Verification items for the finished model (mm, model axes). Give positions to 0.01 mm unless a question says otherwise; leave off trailing zeros. Loops run counter-clockwise (first coordinate to the right, second up) from the corner with the lowest first, then second, coordinate; pieces in that order, holes last. Notation, with made-up numbers: (55, 70) - (80, 70) arc R12 ccw to (80, 76) - close; hole circle Ø8 at (59, 43). An arc over 180 degrees is marked (long way). Answer in a Markdown table with one row per item.
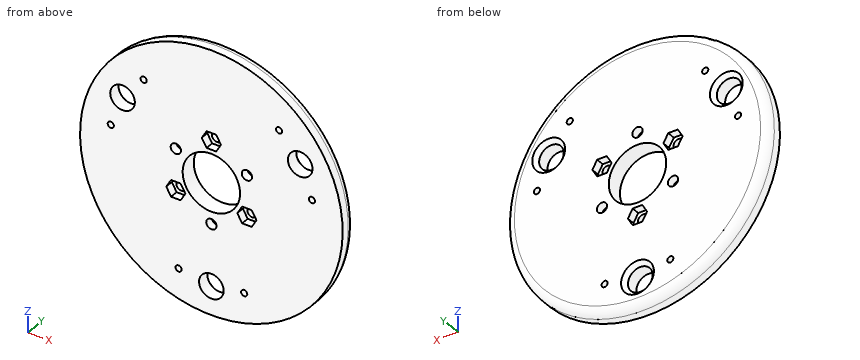
```python
from build123d import *

# Parameters (mm, degrees)
SKETCH_1_R          = 32
SKETCH_1_R_2        = 7
SKETCH_1_R_3        = 3
EXTRUDE_1_DEPTH     = 4
FILLET_1_R          = 2
SKETCH_2_R          = 1.25
CUT_EXTRUDE_1_DEPTH = 46.431266766
CUT_EXTRUDE_2_DEPTH = 2
CUT_EXTRUDE_3_DEPTH = 2
CHAMFER_1_SIZE      = 1
SKETCH_5_R          = 0.75
CUT_EXTRUDE_4_DEPTH = 46.431266766


with BuildPart() as part:
    # Эскиз1 → Бобышка-Вытянуть1 (new body)
    with BuildSketch(Plane(origin=(0, 0, 0), x_dir=(1, 0, 0), z_dir=(0, 1, 0))):
        with Locations(Location((0, 0, 0), (0, 0, 270))):
            Circle(SKETCH_1_R)
        with Locations(Location((0, 0, 0), (0, 0, 270))):
            Circle(SKETCH_1_R_2, mode=Mode.SUBTRACT)
        with Locations(Location((0, 25, 0), (0, 0, 270))):
            Circle(SKETCH_1_R_3, mode=Mode.SUBTRACT)
        with Locations(Location((21.650635095, -12.5, 0), (0, 0, 270))):
            Circle(SKETCH_1_R_3, mode=Mode.SUBTRACT)
        with Locations(Location((-21.650635095, -12.5, 0), (0, 0, 270))):
            Circle(SKETCH_1_R_3, mode=Mode.SUBTRACT)
    extrude(amount=EXTRUDE_1_DEPTH)

    # Скругление1
    fillet_1_edges = [part.edges().sort_by_distance(p)[0] for p in [
        (0, 4, -32),
    ]]
    fillet(fillet_1_edges, radius=FILLET_1_R)

    # Эскиз2 → Вырез-Вытянуть1 (cut, through all)
    with BuildSketch(Plane(origin=(0, 4, 0), x_dir=(1, 0, 0), z_dir=(0, 1, 0))):
        with Locations(Location((0, 10, 0), (0, 0, 270))):
            Circle(SKETCH_2_R)
        with Locations(Location((8.660254038, 5, 0), (0, 0, 270))):
            Circle(SKETCH_2_R)
        with Locations(Location((8.660254038, -5, 0), (0, 0, 270))):
            Circle(SKETCH_2_R)
        with Locations(Location((0, -10, 0), (0, 0, 270))):
            Circle(SKETCH_2_R)
        with Locations(Location((-8.660254038, -5, 0), (0, 0, 270))):
            Circle(SKETCH_2_R)
        with Locations(Location((-8.660254038, 5, 0), (0, 0, 270))):
            Circle(SKETCH_2_R)
    extrude(amount=-CUT_EXTRUDE_1_DEPTH, mode=Mode.SUBTRACT)

    # Эскиз3 → Вырез-Вытянуть2 (cut)
    with BuildSketch(Plane(origin=(0, 4, 0), x_dir=(1, 0, 0), z_dir=(0, 1, 0))):
        Polygon((9.829388333, -7.025), (10.998522628, -5), (9.829388333, -2.975), (7.491119743, -2.975), (6.321985448, -5), (7.491119743, -7.025), align=None)
        Polygon((1.169134295, 7.975), (2.33826859, 10), (1.169134295, 12.025), (-1.169134295, 12.025), (-2.33826859, 10), (-1.169134295, 7.975), align=None)
        Polygon((-10.998522628, -5), (-9.829388333, -7.025), (-7.491119743, -7.025), (-6.321985448, -5), (-7.491119743, -2.975), (-9.829388333, -2.975), align=None)
    extrude(amount=-CUT_EXTRUDE_2_DEPTH, mode=Mode.SUBTRACT)

    # Эскиз4 → Вырез-Вытянуть3 (cut)
    with BuildSketch(Plane.XZ):
        Polygon((7.491119743, -7.025), (9.829388333, -7.025), (10.998522628, -5), (9.829388333, -2.975), (7.491119743, -2.975), (6.321985448, -5), align=None)
        Polygon((-1.169134295, 7.975), (1.169134295, 7.975), (2.33826859, 10), (1.169134295, 12.025), (-1.169134295, 12.025), (-2.33826859, 10), align=None)
        Polygon((-9.829388333, -2.975), (-10.998522628, -5), (-9.829388333, -7.025), (-7.491119743, -7.025), (-6.321985448, -5), (-7.491119743, -2.975), align=None)
    extrude(amount=-CUT_EXTRUDE_3_DEPTH, mode=Mode.SUBTRACT)

    # Фаска1
    chamfer_1_edges = [part.edges().sort_by_distance(p)[0] for p in [
        (21.650635095, 4, 9.5),
        (-21.650635095, 4, 9.5),
        (0, 4, -28),
    ]]
    chamfer(chamfer_1_edges, length=CHAMFER_1_SIZE)

    # Эскиз5 → Вырез-Вытянуть4 (cut, through all)
    with BuildSketch(Plane(origin=(0, 4, 0), x_dir=(1, 0, 0), z_dir=(0, 1, 0))):
        with Locations(Location((8, 23.685438565, 0), (0, 0, 270))):
            Circle(SKETCH_5_R)
        with Locations(Location((-8, 23.685438565, 0), (0, 0, 270))):
            Circle(SKETCH_5_R)
        with Locations(Location((24.512191497, -4.914516052, 0), (0, 0, 270))):
            Circle(SKETCH_5_R)
        with Locations(Location((16.512191497, -18.770922513, 0), (0, 0, 270))):
            Circle(SKETCH_5_R)
        with Locations(Location((-16.512191497, -18.770922513, 0), (0, 0, 270))):
            Circle(SKETCH_5_R)
        with Locations(Location((-24.512191497, -4.914516052, 0), (0, 0, 270))):
            Circle(SKETCH_5_R)
    extrude(amount=-CUT_EXTRUDE_4_DEPTH, mode=Mode.SUBTRACT)


solid = part.part
```
Q1. Thickness scan on line 1 (X direction, y = 0.95, z = 10); line 2 (X direction, y = 0.95, z = 5); line 3 (X direction, y = 2.5, z = 10). Record the ranges inside material, lowest first.
Completed:
| item | result |
|---|---|
| line 1 | -30.4 to -23.31, -19.99 to -2.34, 2.34 to 19.99, 23.31 to 30.4 |
| line 2 | -31.61 to -25.26, -23.77 to -9.91, -7.41 to -4.9, 4.9 to 7.41, 9.91 to 23.77, 25.26 to 31.61 |
| line 3 | -30.33 to -23.31, -19.99 to -1.25, 1.25 to 19.99, 23.31 to 30.33 |
Q2. Sectioned sample at B-B (z = 0). Record the cut outline in (x, y), and give its area (3 significant figures).
Completed:
| item | result |
|---|---|
| outline | (-32, 0) - (-7, 0) - (-7, 4) - (-30, 4) arc R2 ccw to (-32, 2) - close; (7, 0) - (32, 0) - (32, 2) arc R2 ccw to (30, 4) - (7, 4) - close |
| area | 198 mm^2 |
Q3. Sectioned sample at A-A (x = 0). Give the number of separate pieces and of enclosed holes in the cut face, and give its area (3 significant figures).
Completed:
| item | result |
|---|---|
| separate pieces | 5 |
| enclosed holes | 0 |
| area | 147 mm^2 |
Q4. Go/stop test with flat-tipped pins: P1, Ø3, axis at x = 8.66, z = 5, coming from the -Y side; P2, Ø1.5, axis at y = 3, z = -24.5, coming from the -X side; P3, Ø0.6, axis at x = -9, y = 1.5, coming from the +Z side; P4, Ø1, axis at x = -19.5, y = 2, coming from the -Z side. Record where each tip stops, or that it passes through.
Completed:
| item | result |
|---|---|
| P1 | y = 0 |
| P2 | x = -21.19 |
| P3 | z = 30.79 |
| P4 | z = -25.75 |
